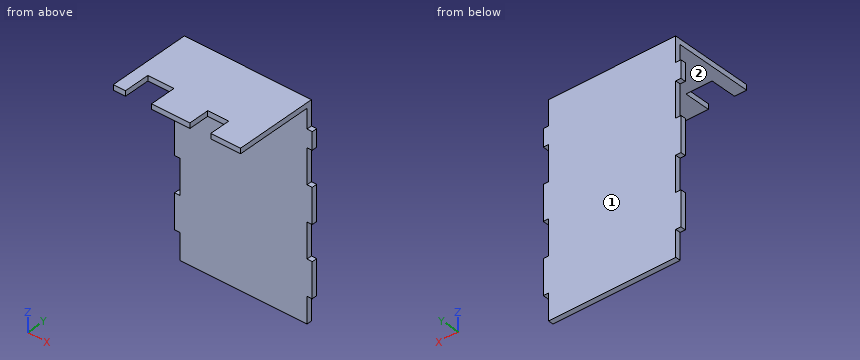
```python
from build123d import *

# Parameters (mm, degrees)
SALIENTE_EXTRUIR1_DEPTH = 3
CROQUIS2_W              = 73.07
CROQUIS2_H              = 3
SALIENTE_EXTRUIR2_DEPTH = 47.72
CROQUIS3_W              = 15
CROQUIS3_H              = 15
CROQUIS3_W_2            = 12
CROQUIS3_H_2            = 12
CORTAR_EXTRUIR1_DEPTH   = 47.72


with BuildPart() as part:
    # Croquis1 → Saliente-Extruir1 (new body)
    with BuildSketch(Plane(origin=(0, 0, 0), x_dir=(1, 0, 0), z_dir=(0, 1, 0))):
        Polygon((29.065596193, -79.884359085), (29.065596193, -82.884359085), (29.065596193, -94.104359085), (-44.004403807, -94.104359085), (-44.004403807, -79.884359085), (-47.004403807, -79.884359085), (-47.004403807, -69.884359085), (-44.004403807, -69.884359085), (-44.004403807, -49.884359085), (-47.004403807, -49.884359085), (-47.004403807, -29.884359085), (-44.004403807, -29.884359085), (-44.004403807, -9.884359085), (-47.004403807, -9.884359085), (-47.004403807, 10.115640915), (-44.004403807, 10.115640915), (-44.004403807, 25.115640915), (29.065596193, 25.115640915), (29.065596193, 10.115640915), (32.065596193, 10.115640915), (32.065596193, -9.884359085), (29.065596193, -9.884359085), (29.065596193, -29.884359085), (32.065596193, -29.884359085), (32.065596193, -49.884359085), (29.065596193, -49.884359085), (29.065596193, -69.884359085), (32.065596193, -69.884359085), (32.065596193, -79.884359085), align=None)
    extrude(amount=SALIENTE_EXTRUIR1_DEPTH)

    # Croquis2 → Saliente-Extruir2 (add)
    with BuildSketch(Plane(origin=(0, 3, 0), x_dir=(1, 0, 0), z_dir=(0, 1, 0))):
        with Locations((-7.469403807, -92.604359085)):
            Rectangle(CROQUIS2_W, CROQUIS2_H)
    extrude(amount=-SALIENTE_EXTRUIR2_DEPTH)

    # Croquis3 → Cortar-Extruir1 (cut)
    with BuildSketch(Plane.XY.offset(94.104359085)):
        with Locations((-29.504403807, -37.22)):
            Rectangle(CROQUIS3_W, CROQUIS3_H)
        with Locations((5.995596193, -38.72)):
            Rectangle(CROQUIS3_W_2, CROQUIS3_H_2)
    extrude(amount=-CORTAR_EXTRUIR1_DEPTH, mode=Mode.SUBTRACT)


solid = part.part
```
The listing builds one solid part. Answer for the finished solid, in the listing's coordinates (mm). Face numbers are marked on the shaded views. A direction names the side the tool comes from. Coordinates: 2 decimals unless noted, no trailing zeros. Write each loop counter-clockwise with the first axis right and the second up, starting at its lowest first coordinate (ties: lowest second). Pieces come first, ordered by that corner, then holes.
Q1. Section B-B, the plane x = -9.5 is taken. Write down the section's boundary in (y, z), then the cut area to 3 significant figures.
Returned:
outline: (-44.72, 91.1) - (0, 91.1) - (0, -25.12) - (3, -25.12) - (3, 94.1) - (-44.72, 94.1) - close
area: 492 mm2
Q2. Section C-C, the plane z = 66 is taken. Write down the section's boundary in (x, y), then the cut area to 3 significant figures.
Returned:
outline: (-44, 0) - (29.07, 0) - (29.07, 3) - (-44, 3) - close
area: 219 mm2
Q3. Section D-D, the plane y = -20 is taken. Write down the section's boundary in (x, z).
Returned:
outline: (-44, 91.1) - (29.07, 91.1) - (29.07, 94.1) - (-44, 94.1) - close
Q4. Section A-A, the plane y = -38 is taken. Write down the section's boundary in (x, z), then the cut area to 3 significant figures.
Returned:
outline: (-44, 91.1) - (-37, 91.1) - (-37, 94.1) - (-44, 94.1) - close; (-22, 91.1) - (0, 91.1) - (0, 94.1) - (-22, 94.1) - close; (12, 91.1) - (29.07, 91.1) - (29.07, 94.1) - (12, 94.1) - close
area: 138 mm2
Q5. Given P1, Ø1, axis at x = -27.5, z = 57.5, coming from the -Y side; P2, Ø3.5, axis at x = 5, z = 93, coming from the -Y side; P3, Ø3.5, axis at y = -37.5, z = 92.5, coming from the +X side; P4, Ø2.5, axis at x = -45, y = 2, coming from the +Z side, each flat-ended and moving along its own axis, determine where each tip first touches the part or whether it passes through.
Returned:
P1: stops at y = 0
P2: stops at y = -32.72
P3: stops at x = 29.07
P4: stops at z = 94.1
Q6. Which of the six approach directions +Z, -Z, +X, -X, +Y, -Y give full straight-line access (tool end or side, diameter ignored) to the marked faces 1 and 2?
Returned:
face 1: +Z, -Z, +X, -X, +Y
face 2: -Z, +X, -X, -Y
Q7. Find the intervals of material crossed by line 1 along Y through (x, z) = (-29.5, 69); line 2 along Z through (x, y) = (-11, -28), in increasing order.
Returned:
line 1: y = 0 to 3
line 2: z = 91.1 to 94.1
